```python
from build123d import *

# Parameters (mm, degrees)
BOSS_EXTRUDE1_DEPTH = 5
BOSS_EXTRUDE2_DEPTH = 15
BOSS_EXTRUDE3_START = 15
BOSS_EXTRUDE3_DEPTH = 15
FILLET2_R           = 5
FILLET3_R           = 5
CUT_EXTRUDE1_DEPTH  = 12
CUT_EXTRUDE2_START  = -12
CUT_EXTRUDE2_DEPTH  = 12
SKETCH11_R          = 2
CUT_EXTRUDE3_DEPTH  = 11


with BuildPart() as part:
    # Sketch4 → Boss-Extrude1 (new body)
    with BuildSketch(Plane(origin=(0, 0, 0), x_dir=(1, 0, 0), z_dir=(0, 1, 0))):
        with BuildLine():
            Line((-57.478675123, 14.203833226), (-47.478675123, 14.203833226))
            ThreePointArc((-47.478675123, 14.203833226), (-32.478675123, -0.796166774), (-17.478675123, 14.203833226))
            Line((-17.478675123, 14.203833226), (2.521324877, 14.203833226))
            ThreePointArc((2.521324877, 14.203833226), (-27.478675123, -15.796166774), (-57.478675123, 14.203833226))
        make_face()
    extrude(amount=BOSS_EXTRUDE1_DEPTH)

    # Sketch5 → Boss-Extrude2 (add)
    with BuildSketch(Plane(origin=(0, 5, 0), x_dir=(1, 0, 0), z_dir=(0, 1, 0))):
        with BuildLine():
            Line((-57.478675123, 14.203833226), (2.521324877, 14.203833226))
            ThreePointArc((2.521324877, 14.203833226), (-27.478675123, -15.796166774), (-57.478675123, 14.203833226))
        make_face()
    extrude(amount=BOSS_EXTRUDE2_DEPTH)

    # Sketch6 → Boss-Extrude3 (add)
    with BuildSketch(Plane.XZ.offset(BOSS_EXTRUDE3_START)):
        with BuildLine():
            Line((2.521324877, -14.203833226), (-57.478675123, -14.203833226))
            ThreePointArc((-57.478675123, -14.203833226), (-27.478675123, 15.796166774), (2.521324877, -14.203833226))
        make_face()
    extrude(amount=-BOSS_EXTRUDE3_DEPTH)

    # Fillet2
    fillet2_edges = [part.edges().sort_by_distance(p)[0] for p in [
        (2.521324877, 2.5, -14.203833226),
    ]]
    fillet(fillet2_edges, radius=FILLET2_R)

    # Fillet3
    fillet3_edges = [part.edges().sort_by_distance(p)[0] for p in [
        (-57.478675123, 2.5, -14.203833226),
    ]]
    fillet(fillet3_edges, radius=FILLET3_R)

    # Sketch8 → Cut-Extrude1 (cut)
    with BuildSketch(Plane(origin=(0, 20, 0), x_dir=(1, 0, 0), z_dir=(0, 1, 0))):
        with BuildLine():
            Line((-51.973572551, 14.203833226), (-2.983777696, 14.203833226))
            ThreePointArc((-2.983777696, 14.203833226), (-27.478675123, -10.291064201), (-51.973572551, 14.203833226))
        make_face()
    extrude(amount=-CUT_EXTRUDE1_DEPTH, mode=Mode.SUBTRACT)

    # Sketch9 → Cut-Extrude2 (cut)
    with BuildSketch(Plane.XZ.offset(15).offset(CUT_EXTRUDE2_START)):
        with BuildLine():
            Line((-51.973572551, -14.203833226), (-2.983777696, -14.203833226))
            ThreePointArc((-2.983777696, -14.203833226), (-27.478675123, 10.291064201), (-51.973572551, -14.203833226))
        make_face()
    extrude(amount=CUT_EXTRUDE2_DEPTH, mode=Mode.SUBTRACT)

    # Sketch11 → Cut-Extrude3 (cut)
    with BuildSketch(Plane.XZ.offset(3)):
        with Locations(Location((-32.478675123, -7.203833226, 0), (0, 0, 270))):
            Circle(SKETCH11_R)
    extrude(amount=-CUT_EXTRUDE3_DEPTH, mode=Mode.SUBTRACT)


solid = part.part
```
The listing builds one solid part. Answer for the finished solid, in the listing's coordinates (mm). A direction names the side the tool comes from. Round coordinates to 2 decimals unless told otherwise and drop trailing zeros. Order: outer loops, then holes, each group sorted by start corner. A loop starts at its lowest first (then second) coordinate and runs counter-clockwise, first axis right, second up. Notation, with made-up numbers: (87, -29.5) - (95, -29.5) arc R21 cw to (95, -15.5) - close; hole circle Ø4 at (89.25, 62.5). An arc over 180 degrees is marked (long way). Put each result on its own line as item: value. Start each with the question number.
(1) Find section D-D (y = -6.5). Give the vertices of the cut face in (x, z), plus the area to 3 significant figures.
(2) Find section C-C (z = 5.5). Give the vertices of the cut face in (x, y), plus the area to 3 significant figures.
(3) Find section A-A (z = -11.5). Give the vertices of the cut face in (x, y).
(4) Find section B-B (x = -19.5). Give the vertices of the cut face in (y, z), plus the area to 3 significant figures.
(5) Determine the mould class of faces 1 (the flat face through (-25, 20, 11)), 2 (the cylindrical face through (-34.25, -1.52, -8.13)), 3 (the cylindrical face through (-55.81, 2.75, -12.41)) for opening direction X: released by +X, released by -X, zero draft, split by the parting line, or undercut.
(6) Given P1, Ø7.5, axis at x = -34, z = -7, coming from the +Y side; P2, Ø1.5, axis at x = -16, y = -3.5, coming from the +Z side; P3, Ø3, axis at x = -32.48, z = -7.2, coming from the -Y side; P4, Ø4, axis at x = -18, z = 0, coming from the -Y side, each flat-ended and moving along its own axis, determine where each tip first touches the part or whether it passes through.
(7) For faces 4 (the flat face through (-27, -15, 11)), 5 (the flat face through (-32, 5, -10)), 6 (the flat face through (-28, -3, -5)), 7 (the cylindrical face through (-34.25, 6.48, -8.13)), 8 (the flat face through (-27, 8, -5)), determine the directions among +Z, -Z, +X, -X, +Y, -Y from which every point of the face is accessible in a straight line to the end or side of a thin tool.
(8) Straight lines are drawn through the part: probe 1 along Y at (x, z) = (-48.5, -8); probe 2 along Y at (x, z) = (-29, -11); probe 3 along X at (y, z) = (-13, 3.25). For each, find the intervals that lie inside material, in ascending order. Write a range as from..to.
Reply:
1. outline: (-56.87, -8.2) arc R5 ccw to (-51.97, -14.2) arc R24.49 cw to (-2.98, -14.2) arc R5 ccw to (1.92, -8.2) arc R30 ccw to start
1. area: 457 mm^2
2. outline: (-50.1, -15) - (-42.03, -15) - (-42.03, -3) - (-12.93, -3) - (-12.93, -15) - (-4.86, -15) - (-4.86, 20) - (-12.93, 20) - (-12.93, 8) - (-42.03, 8) - (-42.03, 20) - (-50.1, 20) - close
2. area: 885 mm^2
3. outline: (-56.42, -15) - (-51.82, -15) - (-51.82, -3) - (-3.13, -3) - (-3.13, -15) - (1.46, -15) - (1.46, 20) - (-3.13, 20) - (-3.13, 8) - (-51.82, 8) - (-51.82, 20) - (-56.42, 20) - close; hole (-47.23, 0) - (-17.72, 0) - (-17.72, 5) - (-47.23, 5) - close
4. outline: (-15, 8.96) - (-3, 8.96) - (-3, -14.2) - (0, -14.2) - (0, -6.68) - (5, -6.68) - (5, -14.2) - (8, -14.2) - (8, 8.96) - (20, 8.96) - (20, 14.72) - (-15, 14.72) - close
4. area: 419 mm^2
5. face 1: zero draft
5. face 2: undercut
5. face 3: released by -X
6. P1: y = 8
6. P2: z = 13.81
6. P3: through
6. P4: y = -3
7. face 4: +Z, -Z, +X, -X, -Y
7. face 5: -Z
7. face 6: -Z, -Y
7. face 7: +Y, -Y
7. face 8: -Z, +Y
8. probe 1: -3..8
8. probe 2: -3..0, 5..8
8. probe 3: -51.88..-44.66, -10.29..-3.08
